Geometry check sheet. Reference: the model listing, model coordinates, mm. A direction names the side the tool comes from. Round coordinates to 2 decimals unless told otherwise and drop trailing zeros. Loops run counter-clockwise (first coordinate to the right, second up) from the corner with the lowest first, then second, coordinate; pieces in that order, holes last. Notation, with made-up numbers: M 73,10 L 104,10 A15 cw 104,25 Z; hole C 49,27.5 d7. An arc over 180 degrees is marked long. Write item = value, one per line.
from build123d import *

# Parameters (mm, degrees)
PAD_DEPTH            = 35
POCKET_DEPTH         = 40.001
POCKET001_DEPTH      = 42.698592
SKETCH021_W          = 20
SKETCH021_H          = 20
POCKET002_DEPTH      = 3
POCKET002_DEPTH_BACK = -2
SKETCH016_R          = 0.5
POCKET003_DEPTH      = 42.698592
SKETCH015_R          = 0.25
POCKET004_DEPTH      = 40.001
POCKET005_DEPTH      = 37.501
PAD001_DEPTH         = 4
SKETCH024_R          = 1.65
POCKET006_DEPTH      = 39.001
SKETCH008_R          = 2.1
POCKET007_DEPTH      = 39.001
SKETCH003_R          = 1.65
POCKET008_DEPTH      = 16
SKETCH004_R          = 1.75
POCKET009_DEPTH      = 13
POCKET010_DEPTH      = 15.5
POCKET010_DEPTH_BACK = -16
SKETCH017_R          = 1.375
POCKET011_DEPTH      = 13.001
CHAMFER_SIZE         = 5


with BuildPart() as part:
    # Sketch → Pad (new body)
    with BuildSketch(Plane.XY):
        with BuildLine():
            Line((20, 20), (20, -20))
            Line((20, -20), (-20, -20))
            Line((-20, -20), (-20, 19.224144))
            ThreePointArc((-5.17104, 20), (-12.746205, 22.68325), (-20, 19.224144))
            Line((-5.17104, 20), (20, 20))
        make_face()
    extrude(amount=-PAD_DEPTH)

    # Sketch001 (on Face3 of Pad) → Pocket (cut, through all)
    with BuildSketch(Plane(origin=(-20, 0, 0), x_dir=(0, -1, 0), z_dir=(-1, 0, 0))):
        Polygon((-10, -8), (10, -8), (10, -16), (5, -16), (5, -18.5), (-5, -18.5), (-5, -16), (-10, -16), align=None)
    extrude(amount=-POCKET_DEPTH, mode=Mode.SUBTRACT)

    # Sketch019 (on Face5 of Pocket) → Pocket001 (cut, through all)
    with BuildSketch(Plane.XZ.offset(20)):
        Polygon((-10, -20.6), (-10, -28.6), (10, -28.6), (10, -20.6), (5, -20.6), (5, -18.1), (-5, -18.1), (-5, -20.6), align=None)
    extrude(amount=-POCKET001_DEPTH, mode=Mode.SUBTRACT)

    # Sketch021 → Pocket002 (cut, two sides)
    with BuildSketch(Plane.XY.offset(-12)) as pocket002_sk:
        Rectangle(SKETCH021_W, SKETCH021_H)
    extrude(amount=-POCKET002_DEPTH, mode=Mode.SUBTRACT)
    extrude(pocket002_sk.sketch, amount=-POCKET002_DEPTH_BACK, mode=Mode.SUBTRACT)

    # Sketch016 (on Face5 of Pocket002) → Pocket003 (cut, through all)
    with BuildSketch(Plane.XZ.offset(20)):
        with Locations((9.983657, -28.602995)):
            Circle(SKETCH016_R)
        with Locations((-10.053121, -28.576208)):
            Circle(SKETCH016_R)
    extrude(amount=-POCKET003_DEPTH, mode=Mode.SUBTRACT)

    # Sketch015 (on Face24 of Pocket003) → Pocket004 (cut, through all)
    with BuildSketch(Plane(origin=(-20, 0, 0), x_dir=(0, -1, 0), z_dir=(-1, 0, 0))):
        with Locations((-10.007711, -7.972068)):
            Circle(SKETCH015_R)
        with Locations((10.132993, -7.972068)):
            Circle(SKETCH015_R)
    extrude(amount=-POCKET004_DEPTH, mode=Mode.SUBTRACT)

    # Sketch025 → Pocket005 (cut, through all)
    with BuildSketch(Plane.XY.offset(2.5)):
        Polygon((10.336529, 29.786797), (28.676373, 3.594785), (36.756538, 10.988299), (24.594908, 30.303831), align=None)
    extrude(amount=-POCKET005_DEPTH, mode=Mode.SUBTRACT)

    # Sketch007 → Pad001 (join)
    with BuildSketch(Plane.XY):
        Polygon((20, -20), (20, 20), (-4.242641, 39.59798), (-39.59798, 4.242641), (-20, -20), align=None)
    extrude(amount=PAD001_DEPTH)

    # Sketch024 → Pocket006 (cut, through all)
    with BuildSketch(Plane.XY.offset(4)):
        with Locations((0.883883, 25.279067)):
            Circle(SKETCH024_R)
        with Locations((-25.279067, -0.883883)):
            Circle(SKETCH024_R)
    extrude(amount=-POCKET006_DEPTH, mode=Mode.SUBTRACT)

    # Sketch008 → Pocket007 (cut, through all)
    with BuildSketch(Plane.XY.offset(4)):
        with Locations((-12.197592, 12.197592)):
            Circle(SKETCH008_R)
    extrude(amount=-POCKET007_DEPTH, mode=Mode.SUBTRACT)

    # Sketch003 → Pocket008 (cut)
    with BuildSketch(Plane.XY.offset(4)):
        with Locations((-8, 7.5)):
            Circle(SKETCH003_R)
        with Locations((8, 7.5)):
            Circle(SKETCH003_R)
        with Locations((-8, -7.5)):
            Circle(SKETCH003_R)
        with Locations((8, -7.5)):
            Circle(SKETCH003_R)
    extrude(amount=-POCKET008_DEPTH, mode=Mode.SUBTRACT)

    # Sketch004 (on Face4 of Pocket008) → Pocket009 (cut)
    with BuildSketch(Plane(origin=(0, 0, -35), x_dir=(1, 0, 0), z_dir=(0, 0, -1))):
        with Locations((-8, 7.5)):
            Circle(SKETCH004_R)
        with Locations((8, 7.5)):
            Circle(SKETCH004_R)
        with Locations((-8, -7.5)):
            Circle(SKETCH004_R)
        with Locations((8, -7.5)):
            Circle(SKETCH004_R)
    extrude(amount=-POCKET009_DEPTH, mode=Mode.SUBTRACT)

    # Sketch022 (on Face6 of Pocket009) → Pocket010 (cut, two sides)
    with BuildSketch(Plane.XY.offset(-16)) as pocket010_sk:
        with BuildLine():
            ThreePointArc((-17.854446, 4.040738), (-16.086679, 4.772971), (-15.354446, 6.540738))
            Line((-15.354446, 6.540738), (-15.354446, 15.354446))
            Line((-15.354446, 15.354446), (-6.540738, 15.354446))
            ThreePointArc((-6.540738, 15.354446), (-4.772971, 16.086679), (-4.040738, 17.854446))
            Line((-4.040738, 22.984446), (-4.040738, 17.854446))
            Line((-22.234446, 22.984446), (-4.040738, 22.984446))
            Line((-22.234446, 4.040738), (-22.234446, 22.984446))
            Line((-22.234446, 4.040738), (-17.854446, 4.040738))
        make_face()
    extrude(amount=-POCKET010_DEPTH, mode=Mode.SUBTRACT)
    extrude(pocket010_sk.sketch, amount=-POCKET010_DEPTH_BACK, mode=Mode.SUBTRACT)

    # Sketch017 → Pocket011 (cut, through all)
    with BuildSketch(Plane.XY.offset(-22)):
        with Locations((-6.540738, 17.854446)):
            Circle(SKETCH017_R)
        with Locations((-17.854446, 6.540738)):
            Circle(SKETCH017_R)
        with Locations((-17.854446, 17.854446)):
            Circle(SKETCH017_R)
    extrude(amount=-POCKET011_DEPTH, mode=Mode.SUBTRACT)

    # Chamfer
    chamfer_edges = [part.edges().sort_by_distance(p)[0] for p in [
        (-4.242641, 39.59798, 2),
        (-39.59798, 4.242641, 2),
    ]]
    chamfer(chamfer_edges, length=CHAMFER_SIZE)


solid = part.part
(1) Depth check by flat-ended pin: pin 1 Ø1.7 at (x, z) = (-19.5, -2.5) entering from +Y; pin 2 Ø2 at (x, y) = (8, 7.5) entering from -Z; pin 3 Ø10 at (y, z) = (-2, -27.5) entering from -X. Enter the tip coordinate at first touch or a pass-through.
Result set:
pin_1 = 4.04
pin_2 = -20.6
pin_3 = -20
(2) Release check for a two-part mould opening along Z. For faces 1 (the cylindrical face through (8.81, 9.05, -31.84)), 2 (the cylindrical face through (-4.79, 16.07, -10.16)) record: released by +Z, released by -Z, zero draft, split by the parting line, or undercut.
Result set:
face_1 = zero draft
face_2 = undercut
(3) Sectioned sample at C-C on x = 4. Record the cut outline in (y, z), then the cut area to 3 significant figures.
Result set:
outline = M -20,-35 L 20,-35 L 20,-28.6 L -20,-28.6 Z; M -20,-18.1 L -5,-18.1 L -5,-16 L -10,-16 L -10,-8.18 A0.25 cw long -9.88,-8 L 9.76,-8 A0.25 cw long 10,-8.22 L 10,-16 L 5,-16 L 5,-18.1 L 20,-18.1 L 20,0 L 32.93,0 L 32.93,4 L -20,4 Z
area = 1,010 mm2
(4) Sectioned sample at B-B on y = -7.5. State how many separate pieces and enclosed holes the cut face has, then the cut area to 3 significant figures.
Result set:
separate_pieces = 5
enclosed_holes = 0
area = 970 mm2
(5) Tool access check on faces 3 (the flat face through (-13, 0, -18.5)), 4 (the cylindrical face through (-5.906, 16.635, -33.226)), 5 (the cylindrical face through (-9.65, 7.57, -1.92)), 6 (the cylindrical face through (-12.63, 22.69, -33.23)). Record the directions out of +Z, -Z, +X, -X, +Y, -Y that give a thin tool (end or side, any length) a straight path to the whole face; none if there is none.
Result set:
face_3 = +X, -X
face_4 = -Z
face_5 = +Z
face_6 = -Z, +Y
(6) Material ranges on line 1 along Y through (x, z) = (-8, -3); line 2 along X through (y, z) = (-7.5, -32); line 3 along Y through (x, z) = (15, -17.5), recorded low to high. Write a range as from..to.
Result set:
line_1 = -20..-9.15, -5.85..5.85, 9.15..15.35
line_2 = -20..-9.75, -6.25..6.25, 9.75..20
line_3 = -20..-5, 5..20
(7) Sectioned sample at A-A on z = -11. Record the cut outline in (x, y).
Result set:
outline = M -20,-20 L 20,-20 L 20,-10 L -20,-10 Z; M -15.35,10 L 20,10 L 20,15.99 L 17.19,20 L -4.04,20 L -4.04,17.85 A2.5 cw -6.54,15.35 L -15.35,15.35 Z; hole C -12.2,12.2 d4.2
(8) Sectioned sample at D-D on z = 1.5. Record the cut outline in (x, y).
Result set:
outline = M -36.45,0.35 L -20,-20 L 20,-20 L 20,20 L -0.35,36.45 L -7.78,36.06 L -36.06,7.78 Z; hole C -25.28,-0.88 d3.3; hole C -12.2,12.2 d4.2; hole C -8,-7.5 d3.3; hole C -8,7.5 d3.3; hole C 0.88,25.28 d3.3; hole C 8,-7.5 d3.3; hole C 8,7.5 d3.3
